Job drawing, mm, ordinate dimensions from the low corner. One solid piece. A direction names the side the tool comes from. Give positions to 0.01 mm unless a question says otherwise; leave off trailing zeros. Order: outer loops, then holes, each group sorted by start corner. A loop starts at its lowest first (then second) coordinate and runs counter-clockwise, first axis right, second up. Notation, with made-up numbers: M -38,3.25 L 7,3.25 A12 cw 7,18.25 Z; hole C 31,-13.5 d4. An arc over 180 degrees is marked long. Use CSV: the item, a comma, the result in double quotes. Start each with the question number.
Item 1: Pin check, flat tip, straight feed: P1, Ø1, axis at x = 3.5, z = 1, coming from the +Y side (3 decimals). Stop position of the tip, or through.
Item 2: Wall check: line 1 along Z through (x, y) = (9.7, 2.5); line 2 along Y through (x, z) = (1.5, 5) (3 decimals); line 3 along Z through (x, y) = (1.5, 0.3). Give the ranges that are in metal, low to high.
Item 3: Band-saw the part on B-B on x = 2. Write the cut outline in (y, z) (3 decimals), plus the area to 3 significant figures.
Item 4: Two-plate mould, pull along Z, no slides. Class the marked faces 3, 4, 5 and 6: pulls with the +Z half, pulls with the -Z half, needs draft (parallel to the pull), parting line crosses it, or undercut.
Item 5: Band-saw the part on D-D on x = 9.7. Write the cut outline in (y, z) (3 decimals), plus the area to 3 significant figures.
Item 6: Band-saw the part on A-A on z = 3. Write the cut outline in (x, y) (3 decimals), plus the area to 3 significant figures.
Item 7: Band-saw the part on C-C on y = 1.4. Write the cut outline in (x, z).
Item 8: Which spindle directions (+Z, -Z, +X, -X, +Y, -Y) get a long thin tool onto all of the face, cutting with end or side? Do the marked faces 1 and 2. Say none if no direction does.
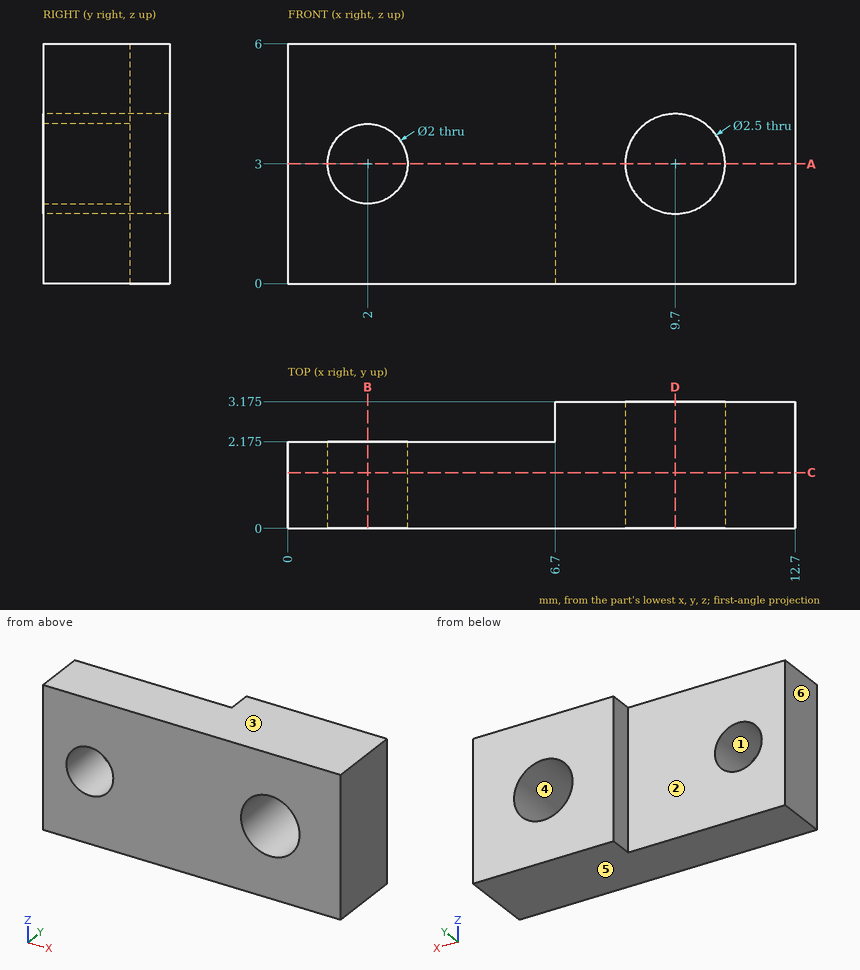
Model answer:
1,P1,"stops at y = 2.175"
2,line 1,"z = 0 to 1.75, 4.25 to 6"
2,line 2,"y = 0 to 2.175"
2,line 3,"z = 0 to 2.13, 3.87 to 6"
3,outline,"M 0,0 L 2.175,0 L 2.175,2 L 0,2 Z; M 0,4 L 2.175,4 L 2.175,6 L 0,6 Z"
3,area,"8.70 mm^2"
4,face 3,"pulls with the +Z half"
4,face 4,"undercut"
4,face 5,"pulls with the -Z half"
4,face 6,"needs draft"
5,outline,"M 0,0 L 3.175,0 L 3.175,1.75 L 0,1.75 Z; M 0,4.25 L 3.175,4.25 L 3.175,6 L 0,6 Z"
5,area,"11.1 mm^2"
6,outline,"M 0,0 L 1,0 L 1,2.175 L 0,2.175 Z; M 3,0 L 8.45,0 L 8.45,3.175 L 6.7,3.175 L 6.7,2.175 L 3,2.175 Z; M 10.95,0 L 12.7,0 L 12.7,3.175 L 10.95,3.175 Z"
6,area,"21.3 mm^2"
7,outline,"M 0,0 L 12.7,0 L 12.7,6 L 0,6 Z; hole C 2,3 d2; hole C 9.7,3 d2.5"
8,face 1,"+Y, -Y"
8,face 2,"+Z, -Z, -X, +Y"
